Verification items for this drawing (mm, ordinates from the low corner). A direction names the side the tool comes from. Give positions to 0.01 mm unless a question says otherwise; leave off trailing zeros. Order: outer loops, then holes, each group sorted by start corner. A loop starts at its lowest first (then second) coordinate and runs counter-clockwise, first axis right, second up. Notation, with made-up numbers: M 28,73 L 66,73 A20 ccw 66,105 Z; hole C 54.25,-31 d10. An arc over 180 degrees is marked long. One line per question, with ' | ' between items. Start each with the question number.
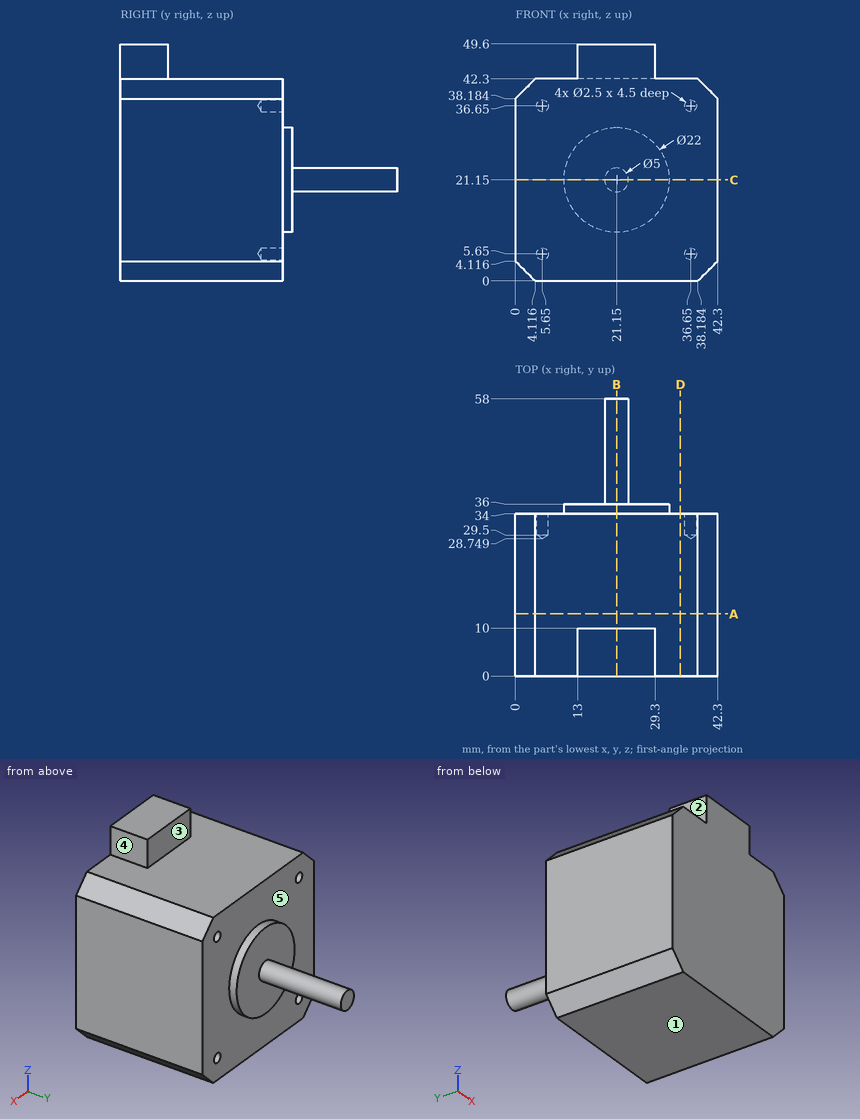
Item 1: Cross-section at B-B, the plane x = 21.15. Record the cut outline in (y, z), plus the area to 3 significant figures.
Item 2: Cross-section at A-A, the plane y = 13. Record the cut outline in (x, z).
Item 3: Set-up check for the marked faces 1, 2, 3, 4 and 5: record each of +Z, -Z, +X, -X, +Y, -Y from which the full face is reachable in a straight line by a thin tool's end or side.
Item 4: Material ranges on line 1 along Z through (x, y) = (36.65, 30.8); line 2 along X through (y, z) = (29.5, 36), recorded low to high.
Item 5: Cross-section at C-C, the plane z = 21.15. Record the cut outline in (x, y), plus the area to 3 significant figures.
Item 6: Cross-section at D-D, the plane x = 34.5. Record the cut outline in (y, z).
Item 7: Depth check by flat-ended pin: pin 1 (6 mm diameter, centred on x = 33.5, z = 35, fed in from +Y); pin 2 (8 mm diameter, centred on y = 41.5, z = 11.5, fed in from -X); pin 3 (8 mm diameter, centred on y = 3.5, z = 44.5, fed in from -X); pin 4 (8 mm diameter, centred on x = 38, y = 16, fed in from +Z). Enter the tip coordinate at first touch or a pass-through.
Outcome:
1) outline: M 0,0 L 34,0 L 34,10.15 L 36,10.15 L 36,18.65 L 58,18.65 L 58,23.65 L 36,23.65 L 36,32.15 L 34,32.15 L 34,42.3 L 10,42.3 L 10,49.6 L 0,49.6 Z | area: 1,670 mm²
2) outline: M 0,4.12 L 4.12,0 L 38.18,0 L 42.3,4.12 L 42.3,38.18 L 38.18,42.3 L 4.12,42.3 L 0,38.18 Z
3) face 1: -Z, +X, -X, +Y, -Y | face 2: +Z, -X, +Y, -Y | face 3: +Z, +X, -X, +Y | face 4: +Z, +X, +Y, -Y | face 5: +Y
4) line 1: z = 0 to 4.4, 6.9 to 35.4, 37.9 to 42.3 | line 2: x = 0 to 4.58, 6.72 to 35.58, 37.72 to 42.3
5) outline: M 0,0 L 42.3,0 L 42.3,34 L 32.15,34 L 32.15,36 L 23.65,36 L 23.65,58 L 18.65,58 L 18.65,36 L 10.15,36 L 10.15,34 L 0,34 Z | area: 1,590 mm²
6) outline: M 0,0 L 34,0 L 34,42.3 L 0,42.3 Z
7) pin 1: stops at y = 34 | pin 2: passes through | pin 3: stops at x = 2.32 | pin 4: stops at z = 42.3
